Here's how the part is built. I have some questions about the finished solid (model axes, mm). Give positions to 0.01 mm unless a question says otherwise; leave off trailing zeros. Write each loop counter-clockwise with the first axis right and the second up, starting at its lowest first coordinate (ties: lowest second). Pieces come first, ordered by that corner, then holes. Notation, with made-up numbers: (63.25, 75.5) -> (72.25, 75.5) arc R34 ccw to (72.25, 111.5) -> close; hole circle Ø9 at (41, -0.5). An arc over 180 degrees is marked (long way). Return JSON: item names as keys, results as strings.
from build123d import *

# Parameters (mm, degrees)
F2_DEPTH = 4.7


with BuildPart() as f2:
    # F1 (on Front) → F2 (new body)
    with BuildSketch(Plane.XZ):
        with BuildLine():
            Line((-92.5, 15), (-92.5, 38))
            ThreePointArc((-92.5, 38), (-93.0857864376, 39.4142135624), (-94.5, 40))
            Line((-94.5, 40), (-102.5, 40))
            ThreePointArc((-102.5, 40), (-106.0355339059, 38.5355339059), (-107.5, 35))
            Line((-107.5, 35), (-107.5, -35))
            ThreePointArc((-107.5, -35), (-106.0355339059, -38.5355339059), (-102.5, -40))
            Line((-102.5, -40), (-92.5, -40))
            Line((-92.5, -40), (-92.5, -20))
            Line((-92.5, -20), (-87.8, -20))
            Line((-87.8, -20), (-87.8, -40))
            Line((-87.8, -40), (87.8, -40))
            Line((87.8, -40), (87.8, -20))
            Line((87.8, -20), (92.5, -20))
            Line((92.5, -20), (92.5, -40))
            Line((92.5, -40), (102.5, -40))
            ThreePointArc((102.5, -40), (106.0355339059, -38.5355339059), (107.5, -35))
            Line((107.5, -35), (107.5, 35))
            ThreePointArc((107.5, 35), (106.0355339059, 38.5355339059), (102.5, 40))
            Line((102.5, 40), (94.5, 40))
            ThreePointArc((94.5, 40), (93.0857864376, 39.4142135624), (92.5, 38))
            Line((92.5, 38), (92.5, 15))
            ThreePointArc((92.5, 15), (88.1066017178, 4.3933982822), (77.5, 0))
            Line((77.5, 0), (-77.5, 0))
            ThreePointArc((-77.5, 0), (-88.1066017178, 4.3933982822), (-92.5, 15))
        make_face()
    extrude(amount=F2_DEPTH)


solid = f2.part
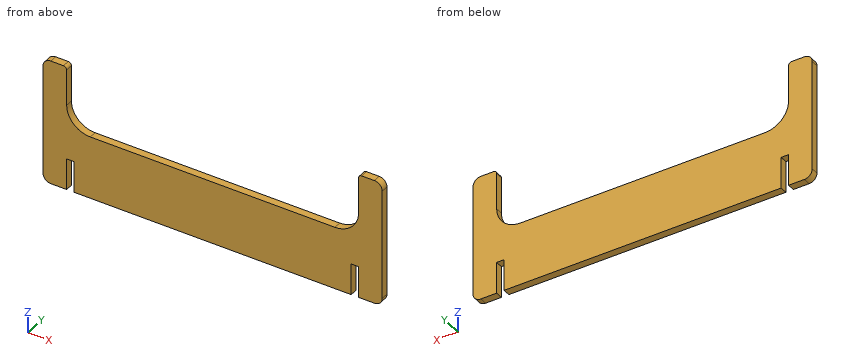
1. Suppose I cut it at C-C, the plane z = 4. List the corners of the cut face in (x, y) for me.
Taken from the geometry:
{"outline": "(-107.5, -4.7) -> (-87.7, -4.7) -> (-87.7, 0) -> (-107.5, 0) -> close; (87.7, -4.7) -> (107.5, -4.7) -> (107.5, 0) -> (87.7, 0) -> close"}
2. Suppose I cut it at B-B, the plane y = -0.75. List the corners of the cut face in (x, z) for me, and give its area (3 significant figures).
Taken from the geometry:
{"outline": "(-107.5, -35) arc R5 ccw to (-102.5, -40) -> (-92.5, -40) -> (-92.5, -20) -> (-87.8, -20) -> (-87.8, -40) -> (87.8, -40) -> (87.8, -20) -> (92.5, -20) -> (92.5, -40) -> (102.5, -40) arc R5 ccw to (107.5, -35) -> (107.5, 35) arc R5 ccw to (102.5, 40) -> (94.5, 40) arc R2 ccw to (92.5, 38) -> (92.5, 15) arc R15 cw to (77.5, 0) -> (-77.5, 0) arc R15 cw to (-92.5, 15) -> (-92.5, 38) arc R2 ccw to (-94.5, 40) -> (-102.5, 40) arc R5 ccw to (-107.5, 35) -> close", "area": "9,690 mm²"}
3. For pin 1 Ø2.5 at (x, y) = (89.5, -1.5) entering from -Z, with a flat end and sliding along its axis, tell me the tip position at first contact or that it passes through.
Taken from the geometry:
{"pin 1": "stops at z = -20"}
4. If I drill on line 1 (X direction, y = -3.95, z = -32); line 2 (X direction, y = -1.85, z = 34); line 3 (Z direction, x = -66, y = -4.4), over which ranges is the centre line in solid material (lowest first)? Write a range as [from, to].
Taken from the geometry:
{"line 1": "x = [-107.5, -92.5], [-87.8, 87.8], [92.5, 107.5]", "line 2": "x = [-107.5, -92.5], [92.5, 107.5]", "line 3": "z = [-40, 0]"}
5. Suppose I cut it at A-A, the plane z = 20. List the corners of the cut face in (x, y) for me.
Taken from the geometry:
{"outline": "(-107.5, -4.7) -> (-92.5, -4.7) -> (-92.5, 0) -> (-107.5, 0) -> close; (92.5, -4.7) -> (107.5, -4.7) -> (107.5, 0) -> (92.5, 0) -> close"}
6. Suppose I cut it at D-D, the plane x = -10. List the corners of the cut face in (y, z) for me.
Taken from the geometry:
{"outline": "(-4.7, -40) -> (0, -40) -> (0, 0) -> (-4.7, 0) -> close"}
